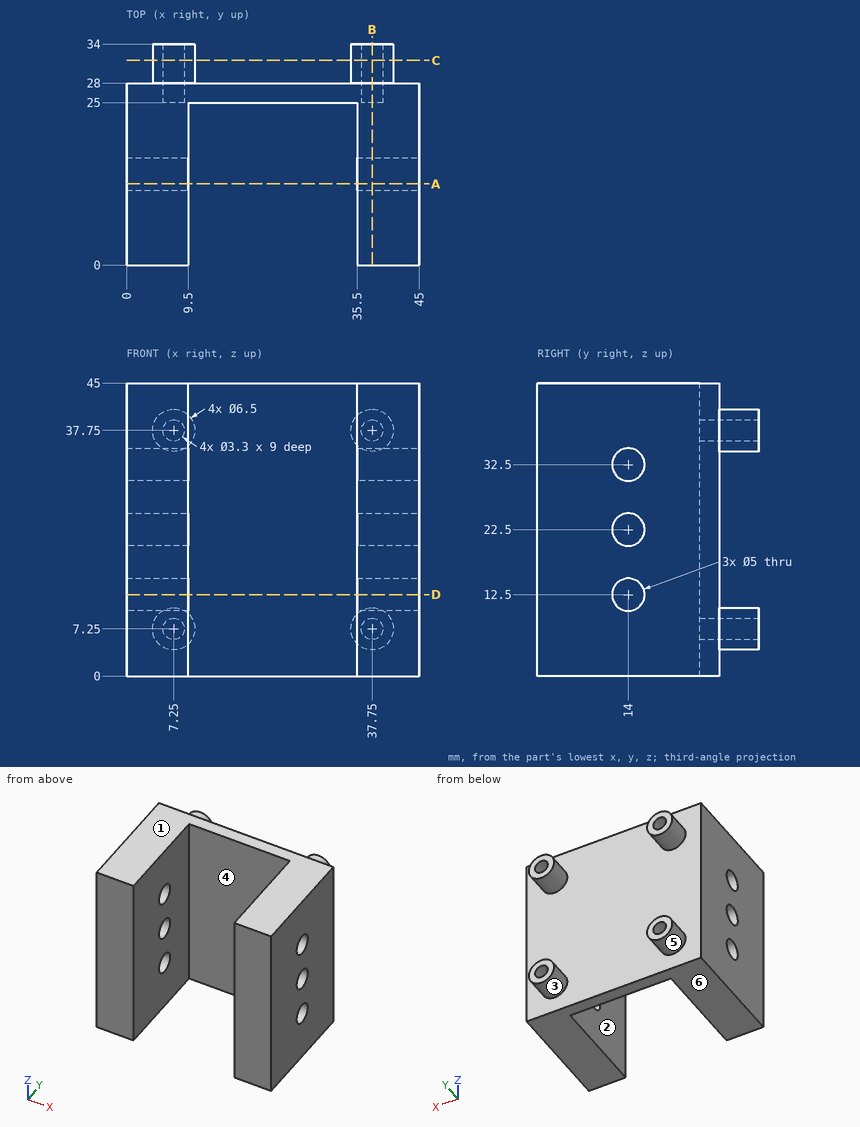
The drawing under review shows one solid part. Ordinate dimensions are in mm from its lowest x, y, z. A direction names the side the tool comes from. Coordinates: 2 decimals unless noted, no trailing zeros. Write each loop counter-clockwise with the first axis right and the second up, starting at its lowest first coordinate (ties: lowest second). Pieces come first, ordered by that corner, then holes. Notation, with made-up numbers: M 45.25,-36.5 L 101.25,-36.5 A21 cw 101.25,-20.5 Z; hole C 20,-17.5 d11. An arc over 180 degrees is marked long. Put each result on its own line as item: value.
1) Add section C-C on y = 31.5. Give the boundary of the cut face in (x, z), then the cut area to 3 significant figures.
Computed:
outline: C 7.25,7.25 d6.5; C 7.25,37.75 d6.5; C 37.75,7.25 d6.5; C 37.75,37.75 d6.5; hole C 7.25,7.25 d3.3; hole C 7.25,37.75 d3.3; hole C 37.75,7.25 d3.3; hole C 37.75,37.75 d3.3
area: 98.5 mm2
2) For the marked faces 4, 5 and 6, list the 3-axis set-ups (+Z, -Z, +X, -X, +Y, -Y) from which the entire face can be reached by the end or side of a thin tool; tool diameter is ignored.
Computed:
face 4: +Z, -Z, -Y
face 5: +Y
face 6: -Z, +X, -X, +Y, -Y
3) Add section D-D on z = 12.5. Give the boundary of the cut face in (x, y), then the cut area to 3 significant figures.
Computed:
outline: M 0,0 L 9.5,0 L 9.5,11.5 L 0,11.5 Z; M 0,16.5 L 9.5,16.5 L 9.5,25 L 35.5,25 L 35.5,16.5 L 45,16.5 L 45,28 L 0,28 Z; M 35.5,0 L 45,0 L 45,11.5 L 35.5,11.5 Z
area: 515 mm2
4) Add section A-A on y = 12.5. State how many separate pieces and enclosed holes the cut face has, then the cut area to 3 significant figures.
Computed:
separate pieces: 8
enclosed holes: 0
area: 627 mm2
5) Add section B-B on x = 37.75. Give the boundary of the cut face in (y, z).
Computed:
outline: M 0,0 L 28,0 L 28,4 L 34,4 L 34,5.6 L 25,5.6 L 25,8.9 L 34,8.9 L 34,10.5 L 28,10.5 L 28,34.5 L 34,34.5 L 34,36.1 L 25,36.1 L 25,39.4 L 34,39.4 L 34,41 L 28,41 L 28,45 L 0,45 Z; hole C 14,12.5 d5; hole C 14,22.5 d5; hole C 14,32.5 d5
6) Wall thickness on probe 1 along X at (y, z) = (30.25, 37.75); probe 2 along X at (y, z) = (27.75, 37.75); probe 3 along X at (y, z) = (1, 16): over which ranges is each line inside the solid? List them lowest first. Write a range as [from, to].
Computed:
probe 1: x = [4, 5.6], [8.9, 10.5], [34.5, 36.1], [39.4, 41]
probe 2: x = [0, 5.6], [8.9, 36.1], [39.4, 45]
probe 3: x = [0, 9.5], [35.5, 45]
7) Draft analysis for pull direction Z (two halves, no side actions). For the marked faces 1, 2 and 3, state which applies: released by +Z, released by -Z, zero draft, split by the parting line, or undercut.
Computed:
face 1: released by +Z
face 2: zero draft
face 3: undercut
8) Clearance check with flat-ended pins moving along their axes: pin 1 Ø1 at (x, z) = (7, 7.5) entering from +Y; pin 2 Ø13 at (x, z) = (24.5, 14) entering from -Y; pin 3 Ø5 at (x, z) = (24, 8) entering from +Y. State where each tip first meets the part, or that it passes through.
Computed:
pin 1: stops at y = 25
pin 2: stops at y = 25
pin 3: stops at y = 28
